from build123d import *

# Parameters (mm, degrees)
F1_DEPTH = 1.5
F0_R     = 2.5
F0_R_2   = 2.55
F0_R_3   = 2.6
F0_R_4   = 2.65
F0_R_5   = 2.7
F2_DEPTH = 12


# Not quite as in the source:
# - a feature names something its author has since deleted; it is built from what else it names


with BuildPart() as f1:
    # F0 (on Top) → F1 (new body)
    with BuildSketch(Plane.XY):
        Polygon((-25.3, 5.5549060926), (-25.3, -8), (25.5, -8), (25.5, 8), (-22.4224738777, 8), (-22.4224738777, 5.5549060926), align=None)
        with BuildLine():
            ThreePointArc((-16.3489727473, -0.6), (-23.7, 0), (-16.3489727473, 0.6))
            Line((-16.3489727473, 0.6), (-13.7016888038, 0.6))
            ThreePointArc((-13.7016888038, 0.6), (-10, 3.75), (-6.2983111962, 0.6))
            Line((-6.2983111962, 0.6), (-3.7523326079, 0.6))
            ThreePointArc((-3.7523326079, 0.6), (0, 3.8), (3.7523326079, 0.6))
            Line((3.7523326079, 0.6), (6.197040626, 0.6))
            ThreePointArc((6.197040626, 0.6), (10, 3.85), (13.802959374, 0.6))
            Line((13.802959374, 0.6), (16.1464302264, 0.6))
            ThreePointArc((16.1464302264, 0.6), (20.3008968951, 3.888375118), (23.9, 0))
            ThreePointArc((23.9, 0), (20.3008968951, -3.888375118), (16.1464302264, -0.6))
            Line((16.1464302264, -0.6), (13.802959374, -0.6))
            ThreePointArc((13.802959374, -0.6), (10, -3.85), (6.197040626, -0.6))
            Line((6.197040626, -0.6), (3.7523326079, -0.6))
            ThreePointArc((3.7523326079, -0.6), (0, -3.8), (-3.7523326079, -0.6))
            Line((-3.7523326079, -0.6), (-6.2983111962, -0.6))
            ThreePointArc((-6.2983111962, -0.6), (-10, -3.75), (-13.7016888038, -0.6))
            Line((-13.7016888038, -0.6), (-16.3489727473, -0.6))
        make_face(mode=Mode.SUBTRACT)
    extrude(amount=F1_DEPTH)

    # F0 (on Top) → F2 (join)
    with BuildSketch(Plane.XY):
        with BuildLine():
            ThreePointArc((-16.3489727473, -0.6), (-16.3122635103, -0.3009976453), (-16.3, 0))
            ThreePointArc((-16.3, 0), (-16.3122635103, 0.3009976453), (-16.3489727473, 0.6))
            ThreePointArc((-16.3489727473, 0.6), (-23.7, 0), (-16.3489727473, -0.6))
        make_face()
        with Locations((-20, 0)):
            Circle(F0_R, mode=Mode.SUBTRACT)
        with BuildLine():
            ThreePointArc((-16.3489727473, 0.6), (-16.3122635103, 0.3009976453), (-16.3, 0))
            ThreePointArc((-16.3, 0), (-16.3122635103, -0.3009976453), (-16.3489727473, -0.6))
            Line((-16.3489727473, -0.6), (-13.7016888038, -0.6))
            ThreePointArc((-13.7016888038, -0.6), (-13.75, 0), (-13.7016888038, 0.6))
            Line((-13.7016888038, 0.6), (-16.3489727473, 0.6))
        make_face()
        with BuildLine():
            ThreePointArc((-6.2983111962, 0.6), (-10, 3.75), (-13.7016888038, 0.6))
            ThreePointArc((-13.7016888038, 0.6), (-13.75, 0), (-13.7016888038, -0.6))
            ThreePointArc((-13.7016888038, -0.6), (-10, -3.75), (-6.2983111962, -0.6))
            ThreePointArc((-6.2983111962, -0.6), (-6.2620973117, -0.3009709171), (-6.25, 0))
            ThreePointArc((-6.25, 0), (-6.2620973117, 0.3009709171), (-6.2983111962, 0.6))
        make_face()
        with Locations((-10, 0)):
            Circle(F0_R_2, mode=Mode.SUBTRACT)
        with BuildLine():
            Line((-3.7523326079, 0.6), (-6.2983111962, 0.6))
            ThreePointArc((-6.2983111962, 0.6), (-6.2620973117, 0.3009709171), (-6.25, 0))
            ThreePointArc((-6.25, 0), (-6.2620973117, -0.3009709171), (-6.2983111962, -0.6))
            Line((-6.2983111962, -0.6), (-3.7523326079, -0.6))
            ThreePointArc((-3.7523326079, -0.6), (-3.8, 0), (-3.7523326079, 0.6))
        make_face()
        with BuildLine():
            ThreePointArc((3.7523326079, 0.6), (0, 3.8), (-3.7523326079, 0.6))
            ThreePointArc((-3.7523326079, 0.6), (-3.8, 0), (-3.7523326079, -0.6))
            ThreePointArc((-3.7523326079, -0.6), (0, -3.8), (3.7523326079, -0.6))
            ThreePointArc((3.7523326079, -0.6), (3.7880644074, -0.3009452526), (3.8, 0))
            ThreePointArc((3.8, 0), (3.7880644074, 0.3009452526), (3.7523326079, 0.6))
        make_face()
        Circle(F0_R_3, mode=Mode.SUBTRACT)
        with BuildLine():
            Line((6.197040626, 0.6), (3.7523326079, 0.6))
            ThreePointArc((3.7523326079, 0.6), (3.7880644074, 0.3009452526), (3.8, 0))
            ThreePointArc((3.8, 0), (3.7880644074, -0.3009452526), (3.7523326079, -0.6))
            Line((3.7523326079, -0.6), (6.197040626, -0.6))
            ThreePointArc((6.197040626, -0.6), (6.15, 0), (6.197040626, 0.6))
        make_face()
        with BuildLine():
            ThreePointArc((13.802959374, 0.6), (10, 3.85), (6.197040626, 0.6))
            ThreePointArc((6.197040626, 0.6), (6.15, 0), (6.197040626, -0.6))
            ThreePointArc((6.197040626, -0.6), (10, -3.85), (13.802959374, -0.6))
            ThreePointArc((13.802959374, -0.6), (13.8382218272, -0.300920596), (13.85, 0))
            ThreePointArc((13.85, 0), (13.8382218272, 0.300920596), (13.802959374, 0.6))
        make_face()
        with Locations((10, 0)):
            Circle(F0_R_4, mode=Mode.SUBTRACT)
        with BuildLine():
            Line((16.1464302264, 0.6), (13.802959374, 0.6))
            ThreePointArc((13.802959374, 0.6), (13.8382218272, 0.300920596), (13.85, 0))
            ThreePointArc((13.85, 0), (13.8382218272, -0.300920596), (13.802959374, -0.6))
            Line((13.802959374, -0.6), (16.1464302264, -0.6))
            ThreePointArc((16.1464302264, -0.6), (16.1, 0), (16.1464302264, 0.6))
        make_face()
        with BuildLine():
            ThreePointArc((23.9, 0), (20.3008968951, 3.888375118), (16.1464302264, 0.6))
            ThreePointArc((16.1464302264, 0.6), (16.1, 0), (16.1464302264, -0.6))
            ThreePointArc((16.1464302264, -0.6), (20.3008968951, -3.888375118), (23.9, 0))
        make_face()
        with Locations((20, 0)):
            Circle(F0_R_5, mode=Mode.SUBTRACT)
    extrude(amount=F2_DEPTH)


solid = f1.part
The model under review builds one solid part; all positions refer to its coordinate system, in mm. A direction names the side the tool comes from. Give positions to 0.01 mm unless a question says otherwise; leave off trailing zeros. Loops run counter-clockwise (first coordinate to the right, second up) from the corner with the lowest first, then second, coordinate; pieces in that order, holes last. Notation, with made-up numbers: (4, 41.5) -> (59, 41.5) arc R17 ccw to (59, 65.5) -> close; hole circle Ø10 at (9.5, -31). An arc over 180 degrees is marked (long way). Answer as a JSON object with one key per item and string values. Group by question number.
Q1. Tool access review of faces 1 (the flat face through (0, -8, 1)), 2 (the flat face through (-24, 5.555, 1)), 3 (the flat face through (-15, 0.6, 7)), 4 (the cylindrical face through (-10.07, -3.75, 6.68)): name each direction out of +Z, -Z, +X, -X, +Y, -Y from which nothing blocks a thin tool from reaching the whole face with its end or side.
Q2. Take a section at A-A (x = 20). Write out the cut boundary in (y, z), plus the area to 3 significant figures.
Q3. Take a section at D-D (y = -5.5). Write out the cut boundary in (x, z).
Q4. Insertion check: pin 1 (8 mm diameter, centred on x = -10, y = 0, fed in from -Z); pin 2 (1.2 mm diameter, centred on x = 15.5, z = 9.5, fed in from -Y); pin 3 (2 mm diameter, centred on x = -4.5, z = 7.5, fed in from -Y); pin 4 (3 mm diameter, centred on x = 0, y = 0, fed in from -Z). Each pin has a flat end and moves straight along its axis. Give the tip position at first contact, or say it passes through.
Q5. Take a section at B-B (z = 4). Write out the cut boundary in (x, y).
Q6. Take a section at C-C (x = -20). Write out the cut boundary in (y, z), plus the area to 3 significant figures.
Q7. Wall thickness on line 1 along Y through (x, z) = (0, 4.75); line 2 along Y through (x, z) = (-10, 4); line 3 along Z through (x, y) = (-18, 3.75): over which ranges is each line inside the solid? List them lowest first.
Answer below:
{
 "1": {"face 1": "+Z, -Z, +X, -X, -Y", "face 2": "+Z, -Z, -X, +Y", "face 3": "+Z, +Y", "face 4": "+Z, -Y"},
 "2": {"outline": "(-8, 0) -> (-2.7, 0) -> (-2.7, 12) -> (-3.9, 12) -> (-3.9, 1.5) -> (-8, 1.5) -> close; (2.7, 0) -> (8, 0) -> (8, 1.5) -> (3.9, 1.5) -> (3.9, 12) -> (2.7, 12) -> close", "area": "41.1 mm2"},
 "3": {"outline": "(-25.3, 0) -> (25.5, 0) -> (25.5, 1.5) -> (-25.3, 1.5) -> close"},
 "4": {"pin 1": "stops at z = 0", "pin 2": "stops at y = -0.6", "pin 3": "stops at y = -1.48", "pin 4": "passes through"},
 "5": {"outline": "(-16.35, -0.6) -> (-13.7, -0.6) arc R3.75 ccw to (-6.3, -0.6) -> (-3.75, -0.6) arc R3.8 ccw to (3.75, -0.6) -> (6.2, -0.6) arc R3.85 ccw to (13.8, -0.6) -> (16.15, -0.6) arc R3.9 ccw (long way) to (16.15, 0.6) -> (13.8, 0.6) arc R3.85 ccw to (6.2, 0.6) -> (3.75, 0.6) arc R3.8 ccw to (-3.75, 0.6) -> (-6.3, 0.6) arc R3.75 ccw to (-13.7, 0.6) -> (-16.35, 0.6) arc R3.7 ccw (long way) to start; hole circle Ø5 at (-20, 0); hole circle Ø5.1 at (-10, 0); hole circle Ø5.2 at (0, 0); hole circle Ø5.3 at (10, 0); hole circle Ø5.4 at (20, 0)"},
 "6": {"outline": "(-8, 0) -> (-2.5, 0) -> (-2.5, 12) -> (-3.7, 12) -> (-3.7, 1.5) -> (-8, 1.5) -> close; (2.5, 0) -> (8, 0) -> (8, 1.5) -> (3.7, 1.5) -> (3.7, 12) -> (2.5, 12) -> close", "area": "41.7 mm2"},
 "7": {"line 1": "y = -3.8 to -2.6, 2.6 to 3.8", "line 2": "y = -3.75 to -2.55, 2.55 to 3.75", "line 3": "z = 0 to 1.5"}
}
